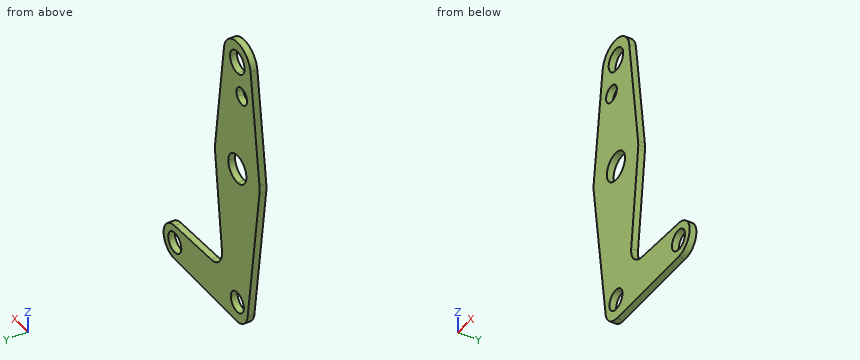
```python
from build123d import *

# Parameters (mm, degrees)
F1_DEPTH = 3.048


with BuildPart() as f1:
    # F0 (on Front) → F1 (new body)
    with BuildSketch(Plane.XZ):
        with BuildLine():
            ThreePointArc((-9.4502929642, 115.490625), (-7.14375, 107.9998046905), (0, 104.775))
            ThreePointArc((0, 104.775), (6.7351920908, 107.5648079092), (9.525, 114.3))
            ThreePointArc((9.525, 114.3), (9.5063048942, 114.896483242), (9.4502929642, 115.490625))
            ThreePointArc((9.4502929642, 115.490625), (0, 123.825), (-9.4502929642, 115.490625))
        make_face()
        with BuildLine():
            ThreePointArc((5.1473989497, 114.3), (3.6397607028, 110.6602392972), (0, 109.1526010503))
            ThreePointArc((0, 109.1526010503), (-3.6397607028, 117.9397607028), (5.1473989497, 114.3))
        make_face(mode=Mode.SUBTRACT)
        with BuildLine():
            ThreePointArc((9.525, 114.3), (6.7351920908, 107.5648079092), (0, 104.775))
            Line((0, 104.775), (0, 102.1312567419))
            ThreePointArc((0, 102.1312567419), (0.4727972806, 101.1250522628), (0.635, 100.0252))
            ThreePointArc((0.635, 100.0252), (0.4727972806, 98.9253477372), (0, 97.9191432581))
            Line((0, 97.9191432581), (0, 79.375))
            ThreePointArc((0, 79.375), (10.5003255158, 75.40625), (15.7504882737, 65.484375))
            Line((15.7504882737, 65.484375), (9.4502929642, 115.490625))
            ThreePointArc((9.4502929642, 115.490625), (9.5063048942, 114.896483242), (9.525, 114.3))
        make_face()
        with BuildLine():
            Line((0, 102.1312567419), (0, 104.775))
            ThreePointArc((0, 104.775), (-7.14375, 107.9998046905), (-9.4502929642, 115.490625))
            Line((-9.4502929642, 115.490625), (-15.7504882737, 65.484375))
            ThreePointArc((-15.7504882737, 65.484375), (-10.5003255158, 75.40625), (0, 79.375))
            Line((0, 79.375), (0, 97.9191432581))
            ThreePointArc((0, 97.9191432581), (-6.985, 100.0252), (0, 102.1312567419))
        make_face()
        with BuildLine():
            ThreePointArc((0, 79.375), (-10.5003255158, 75.40625), (-15.7504882737, 65.484375))
            ThreePointArc((-15.7504882737, 65.484375), (-15.8749354575, 63.4547316886), (-15.7389150973, 61.4258311158))
            ThreePointArc((-15.7389150973, 61.4258311158), (-10.4663315914, 51.5638562333), (0, 47.625))
            Line((0, 47.625), (0, 57.0657531906))
            ThreePointArc((0, 57.0657531906), (-6.4342468094, 63.5), (0, 69.9342468094))
            Line((0, 69.9342468094), (0, 79.375))
        make_face()
        with BuildLine():
            ThreePointArc((15.7504882737, 65.484375), (10.5003255158, 75.40625), (0, 79.375))
            Line((0, 79.375), (0, 69.9342468094))
            ThreePointArc((0, 69.9342468094), (4.5496995508, 68.0496995508), (6.4342468094, 63.5))
            ThreePointArc((6.4342468094, 63.5), (4.5496995508, 58.9503004492), (0, 57.0657531906))
            Line((0, 57.0657531906), (0, 47.625))
            ThreePointArc((0, 47.625), (10.5899458509, 51.6733913621), (15.7786639465, 61.75375))
            ThreePointArc((15.7786639465, 61.75375), (15.8508976899, 62.6255473572), (15.875, 63.5))
            ThreePointArc((15.875, 63.5), (15.8438414904, 64.4941387366), (15.7504882737, 65.484375))
        make_face()
        with BuildLine():
            ThreePointArc((0, 47.625), (-10.4663315914, 51.5638562333), (-15.7389150973, 61.4258311158))
            Line((-15.7389150973, 61.4258311158), (-7.3336929022, -2.3534876791))
            ThreePointArc((-7.3336929022, -2.3534876791), (-4.6020954107, -7.371024327), (0.7890227862, -9.261300353))
            Line((0.7890227862, -9.261300353), (44.5059455788, -7.937302838))
            ThreePointArc((44.5059455788, -7.937302838), (38.85715465, -5.6324050938), (36.5125, 0))
            Line((36.5125, 0), (4.6393582615, 0))
            ThreePointArc((4.6393582615, 0), (-3.2805216871, -3.2805216871), (0, 4.6393582615))
            Line((0, 4.6393582615), (0, 47.625))
        make_face()
        with BuildLine():
            ThreePointArc((15.7786639465, 61.75375), (10.5899458509, 51.6733913621), (0, 47.625))
            Line((0, 47.625), (0, 4.6393582615))
            ThreePointArc((0, 4.6393582615), (3.2805216871, 3.2805216871), (4.6393582615, 0))
            Line((4.6393582615, 0), (36.5125, 0))
            ThreePointArc((36.5125, 0), (38.8978012218, 5.6724769702), (44.6200892857, 7.9356774055))
            Line((44.6200892857, 7.9356774055), (18.5923091973, 8.4935436465))
            ThreePointArc((18.5923091973, 8.4935436465), (12.7834191375, 11.2022395504), (10.8607157214, 17.3164401359))
            Line((10.8607157214, 17.3164401359), (15.7786639465, 61.75375))
        make_face()
        with BuildLine():
            ThreePointArc((36.5125, 0), (38.85715465, -5.6324050938), (44.5059455788, -7.937302838))
            ThreePointArc((44.5059455788, -7.937302838), (50.0824050938, -5.59284535), (52.3875, 0))
            ThreePointArc((52.3875, 0), (50.1224769702, 5.5521987782), (44.6200892857, 7.9356774055))
            ThreePointArc((44.6200892857, 7.9356774055), (38.8978012218, 5.6724769702), (36.5125, 0))
        make_face()
        with BuildLine():
            ThreePointArc((49.088644138, 0), (44.45, -4.638644138), (39.811355862, 0))
            ThreePointArc((39.811355862, 0), (44.45, 4.638644138), (49.088644138, 0))
        make_face(mode=Mode.SUBTRACT)
    extrude(amount=F1_DEPTH)


solid = f1.part
```
The listing builds one solid part. Answer for the finished solid, in the listing's coordinates (mm). Give positions to 0.01 mm unless a question says otherwise; leave off trailing zeros. Order: outer loops, then holes, each group sorted by start corner. A loop starts at its lowest first (then second) coordinate and runs counter-clockwise, first axis right, second up. Notation, with made-up numbers: (8.5, 87.5) -> (30.5, 87.5) arc R22 cw to (30.5, 117.5) -> close; hole circle Ø9 at (31.25, 85.5). An arc over 180 degrees is marked (long way). One line per item, written item: value.
1) Find section A-A, the plane y = -0.75. Count the separate pieces of the cut face and the enclosed holes in it, plus the area to 3 significant figures.
Reported:
separate pieces: 1
enclosed holes: 5
area: 3,440 mm^2
2) Find section B-B, the plane z = 11. Determine the outline of the cut face in (x, y), plus the area to 3 significant figures.
Reported:
outline: (-9.09, -3.05) -> (12.97, -3.05) -> (12.97, 0) -> (-9.09, 0) -> close
area: 67.2 mm^2
3) Find section C-C, the plane x = 20. Determine the outline of the cut face in (y, z).
Reported:
outline: (-3.05, -8.68) -> (0, -8.68) -> (0, 8.46) -> (-3.05, 8.46) -> close
4) Find the intervals of material crossed by line 1 (Z direction, x = -1.5, y = -1.7); line 2 (Z direction, x = 3.5, y = -1); line 3 (X direction, y = -0.3, z = -1.5), in increasing order.
Reported:
line 1: z = -9 to -4.39, 4.39 to 57.24, 69.76 to 96.6, 103.45 to 109.38, 119.22 to 123.71
line 2: z = -9.18 to -3.05, 3.05 to 58.1, 68.9 to 110.53, 118.07 to 123.16
line 3: x = -7.45 to -4.39, 4.39 to 40.06, 48.84 to 52.24
